The model under review builds one solid part; all positions refer to its coordinate system, in mm. Face numbers are marked on the shaded views. Give positions to 0.01 mm unless a question says otherwise; leave off trailing zeros. Loops run counter-clockwise (first coordinate to the right, second up) from the corner with the lowest first, then second, coordinate; pieces in that order, holes last. Notation, with made-up numbers: (14, -20.5) - (41, -20.5) arc R13 ccw to (41, -1.5) - close; hole circle Ø9 at (43, 59). An arc over 180 degrees is marked (long way). Answer as a JSON object with one key per item and string values.
from build123d import *

# Parameters (mm, degrees)
SKETCH1_R           = 15.5
BOSS_EXTRUDE1_DEPTH = 4
CHAMFER1_SIZE       = 3
SKETCH2_R           = 2
CUT_EXTRUDE1_DEPTH  = 4
SKETCH3_R           = 1.5
CUT_EXTRUDE2_DEPTH  = 4
SKETCH4_R           = 1
CUT_EXTRUDE3_DEPTH  = 4


with BuildPart() as part:
    # Sketch1 → Boss-Extrude1 (new body)
    with BuildSketch(Plane(origin=(0, 0, 0), x_dir=(1, 0, 0), z_dir=(0, 1, 0))):
        with Locations(Location((0, 0, 0), (0, 0, 270))):
            Circle(SKETCH1_R)
    extrude(amount=BOSS_EXTRUDE1_DEPTH)

    # Chamfer1
    chamfer1_edges = [part.edges().sort_by_distance(p)[0] for p in [
        (0, 4, -15.5),
    ]]
    chamfer(chamfer1_edges, length=CHAMFER1_SIZE)

    # Sketch2 → Cut-Extrude1 (cut)
    with BuildSketch(Plane(origin=(0, 4, 0), x_dir=(1, 0, 0), z_dir=(0, 1, 0))):
        with Locations(Location((4, 7, 0), (0, 0, 270))):
            Circle(SKETCH2_R)
        with Locations(Location((-4, 7, 0), (0, 0, 270))):
            Circle(SKETCH2_R)
        with Locations(Location((8.062177826, -0.035898385, 0), (0, 0, 270))):
            Circle(SKETCH2_R)
        with Locations(Location((4.062177826, -6.964101615, 0), (0, 0, 270))):
            Circle(SKETCH2_R)
        with Locations(Location((-4.062177826, -6.964101615, 0), (0, 0, 270))):
            Circle(SKETCH2_R)
        with Locations(Location((-8.062177826, -0.035898385, 0), (0, 0, 270))):
            Circle(SKETCH2_R)
    extrude(amount=-CUT_EXTRUDE1_DEPTH, mode=Mode.SUBTRACT)

    # Sketch3 → Cut-Extrude2 (cut)
    with BuildSketch(Plane(origin=(0, 4, 0), x_dir=(1, 0, 0), z_dir=(0, 1, 0))):
        with Locations(Location((0, 0, 0), (0, 0, 270))):
            Circle(SKETCH3_R)
    extrude(amount=-CUT_EXTRUDE2_DEPTH, mode=Mode.SUBTRACT)

    # Sketch4 → Cut-Extrude3 (cut)
    with BuildSketch(Plane(origin=(0, 4, 0), x_dir=(1, 0, 0), z_dir=(0, 1, 0))):
        with Locations(Location((0, 7, 0), (0, 0, 270))):
            Circle(SKETCH4_R)
        with Locations(Location((0, -7, 0), (0, 0, 270))):
            Circle(SKETCH4_R)
    extrude(amount=-CUT_EXTRUDE3_DEPTH, mode=Mode.SUBTRACT)


solid = part.part
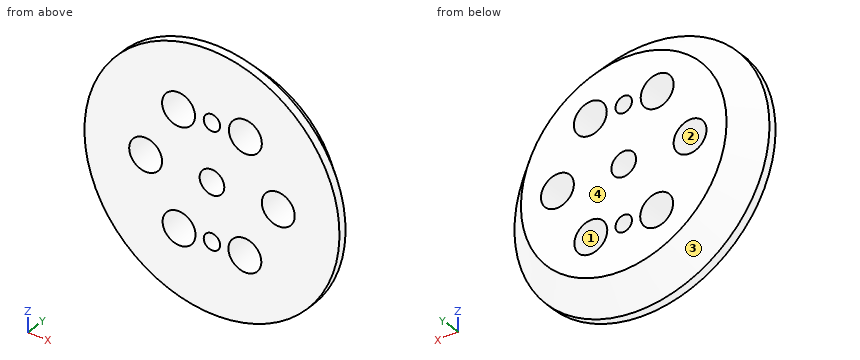
Q1. The part is to be moulded in two halves that separate along X. For the marked faces 1, 2, 3 and 4, say which applies: +X half, -X half, draft (parallel to the pull), parting line (faces both ways), or undercut.
Results:
{"face 1": "undercut", "face 2": "undercut", "face 3": "parting line", "face 4": "draft"}
Q2. To check wall thickness, follow probe 1 along Z at (x, y) = (-0.5, 3.2); probe 2 along X at (y, z) = (2.25, -7); probe 3 along Z at (x, y) = (4.5, 0.65). State the ranges of each line that lie inside material, in increasing order. Write a range as [from, to].
Results:
{"probe 1": "z = [-13.29, -7.87], [-6.13, -1.41], [1.41, 6.13], [7.87, 13.29]", "probe 2": "x = [-12.41, -6], [-2, -1], [1, 2], [6, 12.41]", "probe 3": "z = [-14.83, -8.94], [-5.06, 5.01], [8.92, 14.83]"}
Q3. Consider section B-B, the plane z = 0. State the section outline as (x, y) points.
Results:
{"outline": "(-15.5, 0) - (-10.06, 0) - (-10.06, 4) - (-12.5, 4) - (-15.5, 1) - close; (-6.06, 0) - (-1.5, 0) - (-1.5, 4) - (-6.06, 4) - close; (1.5, 0) - (6.06, 0) - (6.06, 4) - (1.5, 4) - close; (10.06, 0) - (15.5, 0) - (15.5, 1) - (12.5, 4) - (10.06, 4) - close"}
Q4. Consider section A-A, the plane y = 2.4. State how many separate pieces and enclosed holes the cut face has, plus the area to 3 significant figures.
Results:
{"separate pieces": "1", "enclosed holes": "9", "area": "536 mm^2"}
Q5. Clearance check with flat-ended pins moving along their axes: pin 1 Ø2.5 at (x, z) = (4, -7) entering from -Y; pin 2 Ø1 at (x, y) = (-3, 3.5) entering from +Z; pin 3 Ø1 at (y, z) = (1, 5) entering from +X; pin 4 Ø2 at (x, y) = (8.5, 0.5) entering from +Z. State where each tip first meets the part, or that it passes through.
Results:
{"pin 1": "passes through", "pin 2": "stops at z = 13.17", "pin 3": "stops at x = 14.83", "pin 4": "stops at z = 13.56"}
